Input: dimensioned drawing with shaded views. Units: mm. Origin: part minimum x, y, z. Give positions to 0.01 mm unless a question says otherwise; leave off trailing zeros. Write each loop counter-clockwise with the first axis right and the second up, starting at its lowest first coordinate (ties: lowest second). Pieces come first, ordered by that corner, then holes. Notation, with made-up numbers: (5.25, 2) - (55.25, 2) arc R24 cw to (55.25, 14) - close; hole circle Ø6 at (75.25, -30.5). An arc over 180 degrees is marked (long way). Answer as CSV lines item,"result".
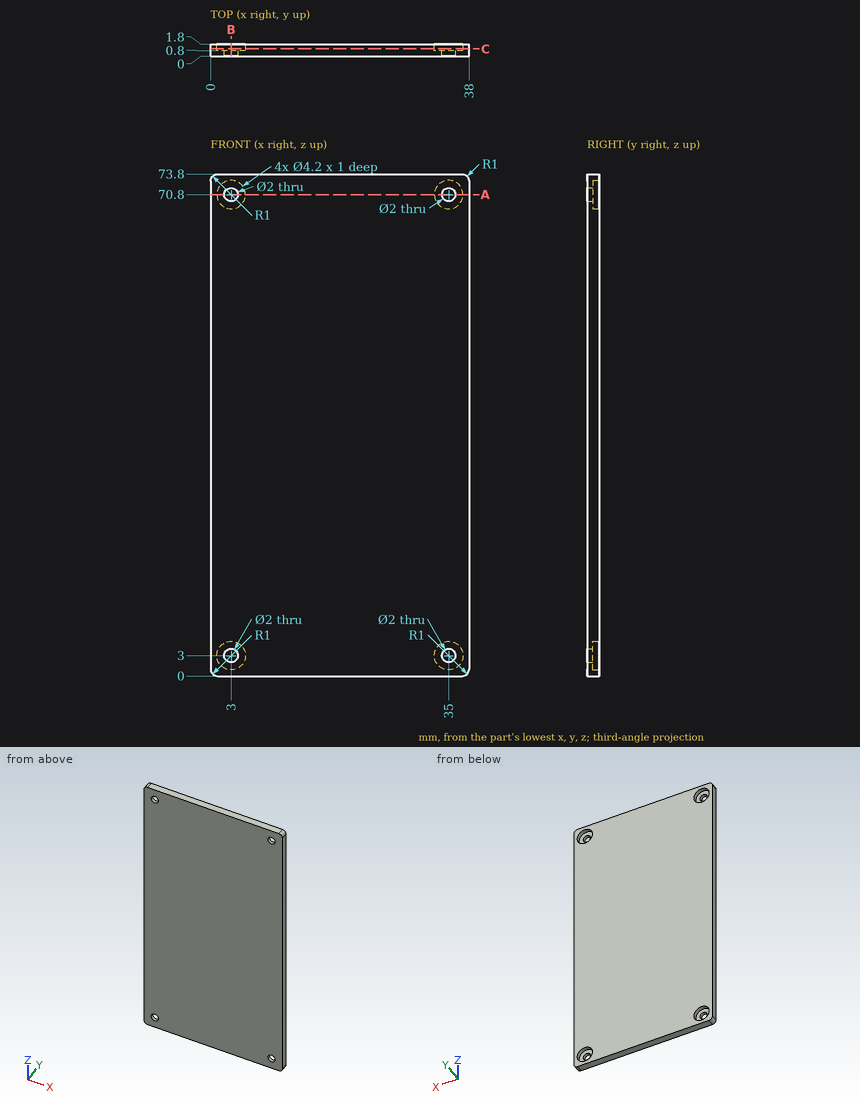
Item 1: Ray query, line 1 (Z direction, x = 35, y = 0.5); line 2 (Z direction, x = 3, y = 1.55); line 3 (X direction, y = 1.1, z = 3). Return the intervals inside material, ascending. Write a range as from..to.
The answers:
line 1,"0..2, 4..69.8, 71.8..73.8"
line 2,"0..0.9, 5.1..68.7, 72.9..73.8"
line 3,"0..0.9, 5.1..32.9, 37.1..38"
Item 2: Cut plane C-C on y = 1.1. Return the cut outline in (x, z), plus the area to 3 significant figures.
The answers:
outline,"(0, 1) arc R1 ccw to (1, 0) - (37, 0) arc R1 ccw to (38, 1) - (38, 72.8) arc R1 ccw to (37, 73.8) - (1, 73.8) arc R1 ccw to (0, 72.8) - close; hole circle Ø4.2 at (3, 3); hole circle Ø4.2 at (3, 70.8); hole circle Ø4.2 at (35, 3); hole circle Ø4.2 at (35, 70.8)"
area,"2,750 mm²"
Item 3: Contact query for flat-ended pins moving along their axis: pin 1 (3.5 mm diameter, centred on x = 3, z = 71, fed in from +Y); pin 2 (6.5 mm diameter, centred on x = 3, z = 70.8, fed in from +Y); pin 3 (1.8 mm diameter, centred on x = 35, z = 3, fed in from -Y). Output: stop coordinate, or through.
The answers:
pin 1,"y = 0.8"
pin 2,"y = 1.8"
pin 3,"through"
Item 4: Cut plane A-A on z = 70.8. Return the cut outline in (x, y), plus the area to 3 significant figures.
The answers:
outline,"(0, 0) - (2, 0) - (2, 0.8) - (0.9, 0.8) - (0.9, 1.8) - (0, 1.8) - close; (4, 0) - (34, 0) - (34, 0.8) - (32.9, 0.8) - (32.9, 1.8) - (5.1, 1.8) - (5.1, 0.8) - (4, 0.8) - close; (36, 0) - (38, 0) - (38, 1.8) - (37.1, 1.8) - (37.1, 0.8) - (36, 0.8) - close"
area,"56.8 mm²"
Item 5: Cut plane B-B on x = 3. Return the cut outline in (y, z), plus the area to 3 significant figures.
The answers:
outline,"(0, 0) - (1.8, 0) - (1.8, 0.9) - (0.8, 0.9) - (0.8, 2) - (0, 2) - close; (0, 4) - (0.8, 4) - (0.8, 5.1) - (1.8, 5.1) - (1.8, 68.7) - (0.8, 68.7) - (0.8, 69.8) - (0, 69.8) - close; (0, 71.8) - (0.8, 71.8) - (0.8, 72.9) - (1.8, 72.9) - (1.8, 73.8) - (0, 73.8) - close"
area,"121 mm²"
